```python
from build123d import *

# Parameters (mm, degrees)
F1_DEPTH  = 381
F2_W      = 609.6
F2_H      = 304.8
F3_DEPTH  = 3.175
F6_DEPTH  = 21.59
F7_R      = 31.75
F8_DEPTH  = 25.4
F9_W      = 304.8
F9_H      = 533.4
F10_DEPTH = 12.7
F10_TAPER = 25
F11_R     = 25.4


with BuildPart() as f1:
    # F0 (on Right) → F1 (new body, symmetric)
    with BuildSketch(Plane.YZ):
        Polygon((-628.65, 0), (0, 0), (0, 762), (-635, 762), (-635, 660.4), (-631.825, 660.4), (-631.825, 657.225), (-635, 657.225), (-635, 113.8153895736), (-628.65, 113.8153895736), align=None)
    extrude(amount=F1_DEPTH, both=True)

    # F2 (on face) → F3 (cut)
    with BuildSketch(Plane.XZ.offset(635)):
        with Locations((0, 381)):
            Rectangle(F2_W, F2_H)
    extrude(amount=-F3_DEPTH, mode=Mode.SUBTRACT)

    # F5 (on offset) → F6 (join, symmetric)
    with BuildSketch(Plane.XY.offset(601.98)):
        Polygon((-330.3532366753, -698.5), (330.3532366753, -698.5), (330.3532366753, -609.3355417252), (298.6032366753, -609.3355417252), (298.6032366753, -679.45), (-298.6032366753, -679.45), (-298.6032366753, -609.3355417252), (-330.3532366753, -609.3355417252), align=None)
    extrude(amount=F6_DEPTH, both=True)

    # F7 (on face) → F8 (join)
    with BuildSketch(Plane.XZ.offset(635)):
        with Locations((-292.1, 707.4763774872)):
            Circle(F7_R)
        with Locations((-165.1, 707.4763774872)):
            Circle(F7_R)
        with Locations((165.1, 707.4763774872)):
            Circle(F7_R)
        with Locations((292.1, 707.4763774872)):
            Circle(F7_R)
    extrude(amount=F8_DEPTH)

    # F9 (on face) → F10 (join)
    with BuildSketch(Plane.XY.offset(762)):
        with Locations((-177.8, -317.5)):
            Rectangle(F9_W, F9_H)
        with Locations((177.8, -317.5)):
            Rectangle(F9_W, F9_H)
    extrude(amount=F10_DEPTH, taper=F10_TAPER)

    # F11
    f11_edges = [f1.edges().sort_by_distance(p)[0] for p in [
        (-327.238946, -581.238946, 768.35),
        (-28.361054, -581.238946, 768.35),
        (28.361054, -581.238946, 768.35),
        (28.361054, -53.761054, 768.35),
        (-327.238946, -53.761054, 768.35),
        (327.238946, -581.238946, 768.35),
        (327.238946, -53.761054, 768.35),
        (-28.361054, -53.761054, 768.35),
    ]]
    fillet(f11_edges, radius=F11_R)


solid = f1.part
```
CAD build for the part. Positions are in the model's coordinates, mm. A direction names the side the tool comes from. Round coordinates to 2 decimals unless told otherwise and drop trailing zeros. Order: outer loops, then holes, each group sorted by start corner. A loop starts at its lowest first (then second) coordinate and runs counter-clockwise, first axis right, second up. Notation, with made-up numbers: (-22.5, 74.5) - (16.5, 74.5) arc R12 ccw to (16.5, 81.5) - close; hole circle Ø4 at (81.25, -39.75). An arc over 180 degrees is marked (long way). Answer in a Markdown table with one row per item. Add a question column.
(1) 3-axis set-ups, long thin cutter, end or side, ignore diameter. For faces 4 (the face through (-330.353, -666, 602)), 5 (the face through (285.22, -647.52, 676.48)), 6 (the face through (292, -660.4, 708)), 7 (the face through (-35.695, -574.254, 769.737)): which of +Z, -Z, +X, -X, +Y, -Y reach the whole face in a straight line?
(2) Band-saw the part on C-C on x = -165.1. List the corners of the cut face in (y, z) (3 decimals).
(3) Probe L1, parallel to Z at x = 291, y = -632 (3 decimals); L2, parallel to Y at x = -53, z = 601; L3, parallel to Y at x = -29, z = 96. List the from-to ranges inside material, lowest first. Write a range as [from, to].
(4) Mould opens along Y. For faces 1 (the face through (165, -660.4, 708)), 2 (the face through (-35.346, -61.095, 769.737)), 3 (the face through (298.603, -657, 602)) say: +Y half, -Y half, draft (parallel to the pull), parting line (faces both ways), or undercut.
(5) Band-saw the part on B-B on z = 494. List the corners of the cut face in (x, y) (3 decimals), and give its area (3 significant figures).
(6) Drop flat-ended pins along their axis: pin 1 Ø3 at (x, z) = (0.5, 688) entering from -Y; pin 2 Ø13 at (x, z) = (-51, 603) entering from +Y; pin 3 Ø13 at (y, z) = (-676, 605.5) entering from -X; pin 4 Ø1.5 at (x, y) = (-163.5, -583) entering from +Z. Give the stop position or say it passes through.
(7) Band-saw the part on A-A on x = -10. List the corners of the cut face in (y, z) (3 decimals).
Data:
| question | item | result |
|---|---|---|
| 1 | face 4 | +Z, -Z, -X, -Y |
| 1 | face 5 | -Y |
| 1 | face 6 | +Z, +X, -X, -Y |
| 1 | face 7 | +Z, -Y |
| 2 | outline | (-698.5, 580.39) - (-679.45, 580.39) - (-679.45, 623.57) - (-698.5, 623.57) - close; (-660.4, 675.726) - (-635, 675.726) - (-635, 660.4) - (-631.825, 660.4) - (-631.825, 657.225) - (-635, 657.225) - (-635, 533.4) - (-631.825, 533.4) - (-631.825, 228.6) - (-635, 228.6) - (-635, 113.815) - (-628.65, 113.815) - (-628.65, 0) - (0, 0) - (0, 762) - (-50.8, 762) - (-56.722, 774.7) - (-578.278, 774.7) - (-584.2, 762) - (-635, 762) - (-635, 739.226) - (-660.4, 739.226) - close |
| 3 | L1 | z = [113.815, 228.6], [533.4, 657.225], [660.4, 762] |
| 3 | L2 | y = [-698.5, -679.45], [-635, 0] |
| 3 | L3 | y = [-628.65, 0] |
| 4 | face 1 | -Y half |
| 4 | face 2 | +Y half |
| 4 | face 3 | undercut |
| 5 | outline | (-381, -635) - (-304.8, -635) - (-304.8, -631.825) - (304.8, -631.825) - (304.8, -635) - (381, -635) - (381, 0) - (-381, 0) - close |
| 5 | area | 482,000 mm^2 |
| 6 | pin 1 | stops at y = -635 |
| 6 | pin 2 | stops at y = 0 |
| 6 | pin 3 | stops at x = -330.35 |
| 6 | pin 4 | stops at z = 766.18 |
| 7 | outline | (-698.5, 580.39) - (-679.45, 580.39) - (-679.45, 623.57) - (-698.5, 623.57) - close; (-635, 113.815) - (-628.65, 113.815) - (-628.65, 0) - (0, 0) - (0, 762) - (-635, 762) - (-635, 660.4) - (-631.825, 660.4) - (-631.825, 657.225) - (-635, 657.225) - (-635, 533.4) - (-631.825, 533.4) - (-631.825, 228.6) - (-635, 228.6) - close |
